```python
from build123d import *

# Parameters (mm, degrees)
SKETCH_1_W      = 76.5
SKETCH_1_H      = 52
EXTRUDE_1_DEPTH = 2
SKETCH_2_W      = 72.5
SKETCH_2_H      = 48
SKETCH_2_W_2    = 68.5
SKETCH_2_H_2    = 44
EXTRUDE_2_DEPTH = 4
FILLET_1_R      = 1


with BuildPart() as part:
    # Эскиз1 → Бобышка-Вытянуть1 (new body)
    with BuildSketch(Plane(origin=(0, 0, 0), x_dir=(1, 0, 0), z_dir=(0, 1, 0))):
        with Locations((-16.564317774, 1.63491921)):
            Rectangle(SKETCH_1_W, SKETCH_1_H)
    extrude(amount=EXTRUDE_1_DEPTH)

    # Эскиз2 → Бобышка-Вытянуть2 (add)
    with BuildSketch(Plane(origin=(0, 2, 0), x_dir=(1, 0, 0), z_dir=(0, 1, 0))):
        with Locations((-16.564317774, 1.63491921)):
            Rectangle(SKETCH_2_W, SKETCH_2_H)
        with Locations((-16.564317774, 1.63491921)):
            Rectangle(SKETCH_2_W_2, SKETCH_2_H_2, mode=Mode.SUBTRACT)
    extrude(amount=EXTRUDE_2_DEPTH)

    # Скругление1
    fillet_1_edges = [part.edges().sort_by_distance(p)[0] for p in [
        (-50.814317774, 2, -1.63491921),
        (-16.564317774, 2, 20.36508079),
        (17.685682226, 2, -1.63491921),
        (-16.564317774, 2, -23.63491921),
    ]]
    fillet(fillet_1_edges, radius=FILLET_1_R)


solid = part.part
```
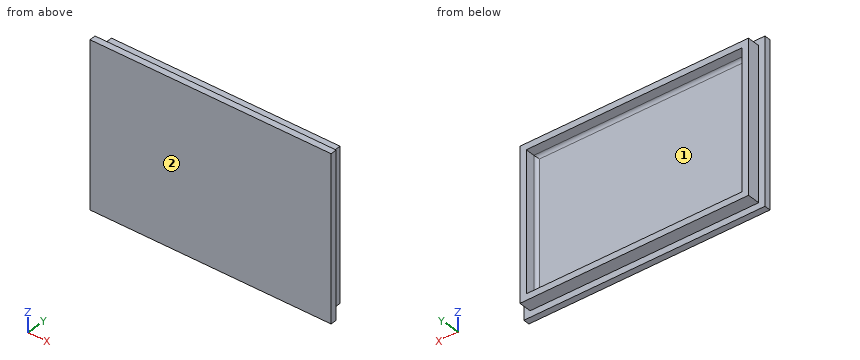
The model under review builds one solid part; all positions refer to its coordinate system, in mm. Face numbers are marked on the shaded views. Round coordinates to 2 decimals unless told otherwise and drop trailing zeros. Loops run counter-clockwise (first coordinate to the right, second up) from the corner with the lowest first, then second, coordinate; pieces in that order, holes last. Notation, with made-up numbers: (44, 54.5) -> (100, 54.5) arc R30 cw to (100, 88.5) -> close; hole circle Ø11 at (43, 32.5). An arc over 180 degrees is marked (long way). Answer as a JSON object with one key per item and string values. Group by question number.
1) We need section C-C on z = 12. Write out the cut boundary in (x, y), then the cut area to 3 significant figures.
2) We need section A-A on y = 4.75. Write out the cut boundary in (x, z).
3) For pin 1 Ø3.5 at (x, y) = (-18, 5) entering from +Z; pin 2 Ø3 at (y, z) = (4, 3.5) entering from -X; pin 3 Ø3.5 at (x, y) = (-23.5, 4) entering from -Z, all flat-tipped, find the tip position at first contact; note any pin that passes through.
4) For line 1 (X direction, y = 4.8, z = 6); line 2 (Z direction, x = -0.5, y = 3.25); line 3 (Y direction, x = -38.5, z = 6), list the stretches that pass through material, from the lowest coordinate up. Write a range as [from, to].
5) We need section B-B on x = 7.5. Write out the cut boundary in (y, z), then the cut area to 3 significant figures.
6) Mouldability with a two-part tool opening along X and no side actions: class the marked faces 1 and 2 as released by +X, released by -X, zero draft, split by the parting line, or undercut.
Result set:
{
 "1": {"outline": "(-54.81, 0) -> (21.69, 0) -> (21.69, 2) -> (19.69, 2) -> (19.69, 6) -> (17.69, 6) -> (17.69, 3) arc R1 cw to (16.69, 2) -> (-49.81, 2) arc R1 cw to (-50.81, 3) -> (-50.81, 6) -> (-52.81, 6) -> (-52.81, 2) -> (-54.81, 2) -> close", "area": "169 mm²"},
 "2": {"outline": "(-52.81, -25.63) -> (19.69, -25.63) -> (19.69, 22.37) -> (-52.81, 22.37) -> close; hole (-50.81, -23.63) -> (17.69, -23.63) -> (17.69, 20.37) -> (-50.81, 20.37) -> close"},
 "3": {"pin 1": "z = 22.37", "pin 2": "x = -52.81", "pin 3": "z = -25.63"},
 "4": {"line 1": "[-52.81, -50.81], [17.69, 19.69]", "line 2": "[-25.63, -23.63], [20.37, 22.37]", "line 3": "[0, 2]"},
 "5": {"outline": "(0, -27.63) -> (2, -27.63) -> (2, -25.63) -> (6, -25.63) -> (6, -23.63) -> (3, -23.63) arc R1 cw to (2, -22.63) -> (2, 19.37) arc R1 cw to (3, 20.37) -> (6, 20.37) -> (6, 22.37) -> (2, 22.37) -> (2, 24.37) -> (0, 24.37) -> close", "area": "120 mm²"},
 "6": {"face 1": "undercut", "face 2": "zero draft"}
}
